Geometry check sheet. Reference: drawing and pictorial views, mm from the part's lowest x, y, z. Give positions to 0.01 mm unless a question says otherwise; leave off trailing zeros. Loops run counter-clockwise (first coordinate to the right, second up) from the corner with the lowest first, then second, coordinate; pieces in that order, holes last. Notation, with made-up numbers: M 22.25,61 L 50.25,61 A14 ccw 50.25,72 Z; hole C 4,12 d2. An arc over 180 degrees is marked long. One line per question, with ' | ' between items. Start each with the question number.
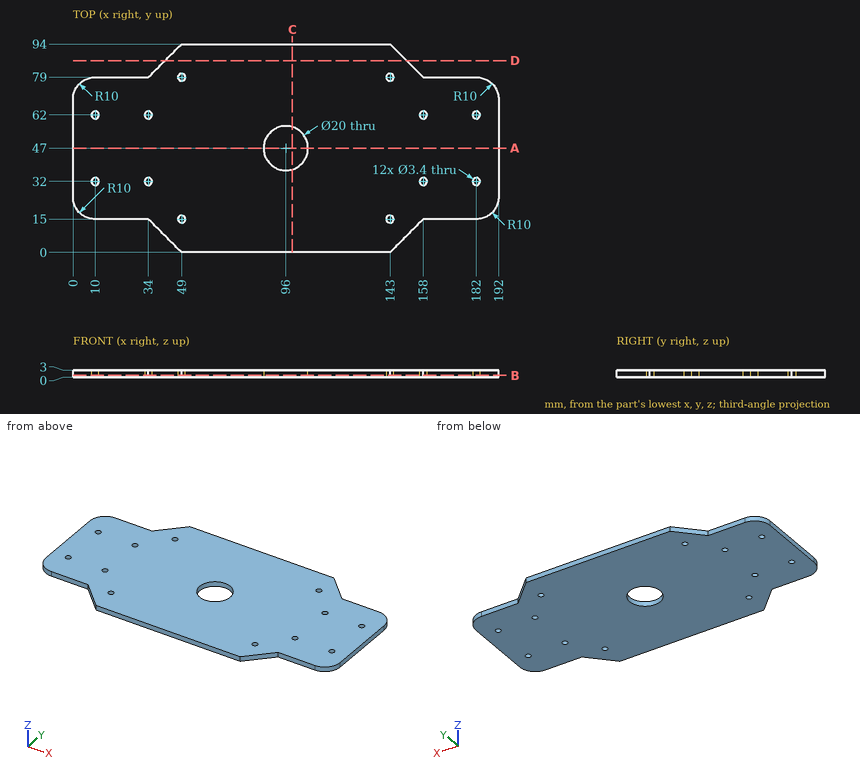
Q1. Material ranges on probe 1 along X at (y, z) = (32, 1.4); probe 2 along Y at (x, z) = (143, 0.7); probe 3 along X at (y, z) = (30.5, 1.45), recorded low to high. Write a range as from..to.
Q2. Depth check by flat-ended pin: P1, Ø10, axis at x = 48.5, y = 11, coming from the -Z side; P2, Ø2, axis at x = 10, y = 62, coming from the +Z side; P3, Ø1.5, axis at x = 22.5, z = 2, coming from the +Y side. Enter the tip coordinate at first touch or a pass-through.
Q3. Cross-section at D-D (y = 86.5). Record the cut outline in (x, z).
Q4. Cross-section at C-C (x = 99). Record the cut outline in (y, z).
Q5. Cross-section at B-B (z = 0.8). State how many separate pieces and enclosed holes the cut face has, and give its area (3 significant figures).
Q6. Cross-section at A-A (y = 47). Record the cut outline in (x, z), and give its area (3 significant figures).
Solved:
1) probe 1: x = 0..8.3, 11.7..32.3, 35.7..156.3, 159.7..180.3, 183.7..192 | probe 2: y = 0..13.3, 16.7..77.3, 80.7..94 | probe 3: x = 0..9.2, 10.8..33.2, 34.8..157.2, 158.8..181.2, 182.8..192
2) P1: stops at z = 0 | P2: passes through | P3: stops at y = 79
3) outline: M 41.5,0 L 150.5,0 L 150.5,3 L 41.5,3 Z
4) outline: M 0,0 L 37.46,0 L 37.46,3 L 0,3 Z; M 56.54,0 L 94,0 L 94,3 L 56.54,3 Z
5) separate pieces: 1 | enclosed holes: 13 | area: 15,000 mm²
6) outline: M 0,0 L 86,0 L 86,3 L 0,3 Z; M 106,0 L 192,0 L 192,3 L 106,3 Z | area: 516 mm²
